The listing builds one solid part. Answer for the finished solid, in the listing's coordinates (mm). A direction names the side the tool comes from. Give positions to 0.01 mm unless a question says otherwise; leave off trailing zeros. Loops run counter-clockwise (first coordinate to the right, second up) from the corner with the lowest first, then second, coordinate; pieces in that order, holes last. Notation, with made-up numbers: (30, 22) - (50, 22) arc R32 ccw to (50, 54) - close; hole circle Ø6 at (16, 9). An arc over 180 degrees is marked (long way). Write each question's results on one line, items separated by ' | '.
from build123d import *

# Parameters (mm, degrees)
EXTRUDE_1_DEPTH     = 3.5
SKETCH_4_R          = 2
CUT_EXTRUDE_1_DEPTH = 85.167986788
SKETCH_4_3_R        = 2.5
SKETCH_4_3_R_2      = 2
CUT_EXTRUDE_2_DEPTH = 2.5
SKETCH_4_5_R        = 3
SKETCH_4_5_R_2      = 2.5
CUT_EXTRUDE_4_DEPTH = 0.5
EXTRUDE_START       = 6
SKETCH_5_R          = 4
EXTRUDE_2_DEPTH     = 6
SKETCH_6_R          = 2
CUT_EXTRUDE_5_DEPTH = 85.630077396
SKETCH_6_3_R        = 2.5
SKETCH_6_3_R_2      = 2
CUT_EXTRUDE_6_DEPTH = 2.5
SKETCH_6_4_R        = 3
SKETCH_6_4_R_2      = 2.5
CUT_EXTRUDE_7_DEPTH = 0.5
CUT_EXTRUDE_START   = -2.5
SKETCH_7_R          = 2.5
CUT_EXTRUDE_8_DEPTH = 2.5
CUT_EXTRUDE_START_2 = -0.5
SKETCH_7_3_R        = 3
SKETCH_7_3_R_2      = 2.5
CUT_EXTRUDE_9_DEPTH = 0.5


with BuildPart() as part:
    # Sketch 3 → Extrude 1 (new body)
    with BuildSketch(Plane.XY):
        with BuildLine():
            Line((0, 4), (80, 4))
            ThreePointArc((80, 4), (84, 0), (80, -4))
            Line((80, -4), (0, -4))
            ThreePointArc((0, -4), (-4, 0), (0, 4))
        make_face()
    extrude(amount=EXTRUDE_1_DEPTH)

    # Sketch 4 → Cut-Extrude 1 (cut, through all)
    with BuildSketch(Plane(origin=(0, 0, 0), x_dir=(-1, 0, 0), z_dir=(0, 0, -1))):
        Circle(SKETCH_4_R)
    extrude(amount=-CUT_EXTRUDE_1_DEPTH, mode=Mode.SUBTRACT)

    # Sketch 4_3 → Cut-Extrude 2 (cut)
    with BuildSketch(Plane(origin=(0, 0, 0), x_dir=(-1, 0, 0), z_dir=(0, 0, -1))):
        Circle(SKETCH_4_3_R)
        Circle(SKETCH_4_3_R_2, mode=Mode.SUBTRACT)
    extrude(amount=-CUT_EXTRUDE_2_DEPTH, mode=Mode.SUBTRACT)

    # Sketch 4_5 → Cut-Extrude 4 (cut)
    with BuildSketch(Plane(origin=(0, 0, 0), x_dir=(-1, 0, 0), z_dir=(0, 0, -1))):
        Circle(SKETCH_4_5_R)
        Circle(SKETCH_4_5_R_2, mode=Mode.SUBTRACT)
    extrude(amount=-CUT_EXTRUDE_4_DEPTH, mode=Mode.SUBTRACT)

    # Sketch 5 → Extrude 2 (add)
    with BuildSketch(Plane(origin=(0, 0, 0), x_dir=(-1, 0, 0), z_dir=(0, 0, -1)).offset(EXTRUDE_START)):
        with Locations((-80, 0)):
            Circle(SKETCH_5_R)
    extrude(amount=-EXTRUDE_2_DEPTH)

    # Sketch 6 → Cut-Extrude 5 (cut, through all)
    with BuildSketch(Plane(origin=(0, 0, -6), x_dir=(-1, 0, 0), z_dir=(0, 0, -1))):
        with Locations((-80, 0)):
            Circle(SKETCH_6_R)
    extrude(amount=-CUT_EXTRUDE_5_DEPTH, mode=Mode.SUBTRACT)

    # Sketch 6_3 → Cut-Extrude 6 (cut)
    with BuildSketch(Plane(origin=(0, 0, -6), x_dir=(-1, 0, 0), z_dir=(0, 0, -1))):
        with Locations((-80, 0)):
            Circle(SKETCH_6_3_R)
        with Locations((-80, 0)):
            Circle(SKETCH_6_3_R_2, mode=Mode.SUBTRACT)
    extrude(amount=-CUT_EXTRUDE_6_DEPTH, mode=Mode.SUBTRACT)

    # Sketch 6_4 → Cut-Extrude 7 (cut)
    with BuildSketch(Plane(origin=(0, 0, -6), x_dir=(-1, 0, 0), z_dir=(0, 0, -1))):
        with Locations((-80, 0)):
            Circle(SKETCH_6_4_R)
        with Locations((-80, 0)):
            Circle(SKETCH_6_4_R_2, mode=Mode.SUBTRACT)
    extrude(amount=-CUT_EXTRUDE_7_DEPTH, mode=Mode.SUBTRACT)

    # Sketch 7 → Cut-Extrude 8 (cut)
    with BuildSketch(Plane.XY.offset(3.5).offset(CUT_EXTRUDE_START)):
        with Locations(Location((80, 0, 0), (0, 0, 180))):
            Circle(SKETCH_7_R)
    extrude(amount=CUT_EXTRUDE_8_DEPTH, mode=Mode.SUBTRACT)

    # Sketch 7_3 → Cut-Extrude 9 (cut)
    with BuildSketch(Plane.XY.offset(3.5).offset(CUT_EXTRUDE_START_2)):
        with Locations(Location((80, 0, 0), (0, 0, 180))):
            Circle(SKETCH_7_3_R)
        with Locations((80, 0)):
            Circle(SKETCH_7_3_R_2, mode=Mode.SUBTRACT)
    extrude(amount=CUT_EXTRUDE_9_DEPTH, mode=Mode.SUBTRACT)


solid = part.part
Item 1: Flat-ended cylindrical pins translate along their axes: P1, Ø1.5, axis at y = -2.5, z = 2.5, coming from the -X side; P2, Ø2, axis at x = 57.5, y = 0.5, coming from the -Z side; P3, Ø2.5, axis at x = -1, y = -1, coming from the -Z side. Find the tip coordinate at first contact, or state that the pin passes through.
Values found:
P1: stops at x = -3.6 | P2: stops at z = 0 | P3: stops at z = 0.5
Item 2: A cutting plane is placed at C-C, the plane x = 11.5. Determine the outline of the cut face in (y, z), plus the area to 3 significant figures.
Values found:
outline: (-4, 0) - (4, 0) - (4, 3.5) - (-4, 3.5) - close | area: 28.0 mm²
Item 3: A cutting plane is placed at A-A, the plane z = -1.5. Determine the outline of the cut face in (x, y), plus the area to 3 significant figures.
Values found:
outline: circle Ø8 at (80, 0); hole circle Ø4 at (80, 0) | area: 37.7 mm²
Item 4: For a pull along Y with two mould halves and no side action, classify faces 1 (the face through (-4, 0, 2)), 2 (the face through (39, 4, 2)), 3 (the face through (3, 0.1, 0.2)) as released by +Y, released by -Y, zero draft, split by the parting line, or undercut.
Values found:
face 1: split by the parting line | face 2: released by +Y | face 3: undercut
Item 5: Find the intervals of material crossed by line 1 along Y through (x, z) = (80, 2.6); line 2 along Y through (x, z) = (0, 2.7); line 3 along Z through (x, y) = (12.5, -3.5), in increasing order. Write a range as [from, to].
Values found:
line 1: y = [-4, -2.5], [2.5, 4] | line 2: y = [-4, -2], [2, 4] | line 3: z = [0, 3.5]
Item 6: For faces 4 (the face through (83, -0.1, 3.2)), 5 (the face through (78.092, 0.601, -1.281)), 6 (the face through (82.5, 0.1, -4.5)), determine the directions among +Z, -Z, +X, -X, +Y, -Y from which every point of the face is accessible in a straight line to the end or side of a thin tool.
Values found:
face 4: +Z | face 5: +Z, -Z | face 6: -Z
Item 7: A cutting plane is placed at B-B, the plane y = 0. Count the separate pieces of the cut face and the enclosed holes in it, plus the area to 3 significant figures.
Values found:
separate pieces: 3 | enclosed holes: 0 | area: 295 mm²
